Geometry: final body of the model. Coordinates: model frame, mm. Give positions to 0.01 mm unless a question says otherwise; leave off trailing zeros. Write each loop counter-clockwise with the first axis right and the second up, starting at its lowest first coordinate (ties: lowest second). Pieces come first, ordered by that corner, then holes.
Q1. Line query: L1, parallel to Y at x = 2.5, z = 261.5; L2, parallel to Z at x = 1, y = 2; L3, parallel to Z at x = 0.5, y = 1.5. Output: solid intervals per line, ascending.
Q2. Cut plane D-D on y = 71. Return the cut outline in (x, z).
Q3. Cut plane A-A on z = -257. Return the cut outline in (x, y).
Q4. Cut plane B-B on y = 13.5. Return the cut outline in (x, z), plus the area to 3 significant figures.
Q5. Cut plane C-C on x = 3.5. Count the separate pieces of the cut face and the enclosed holes in it, plus the area to 3 significant figures.
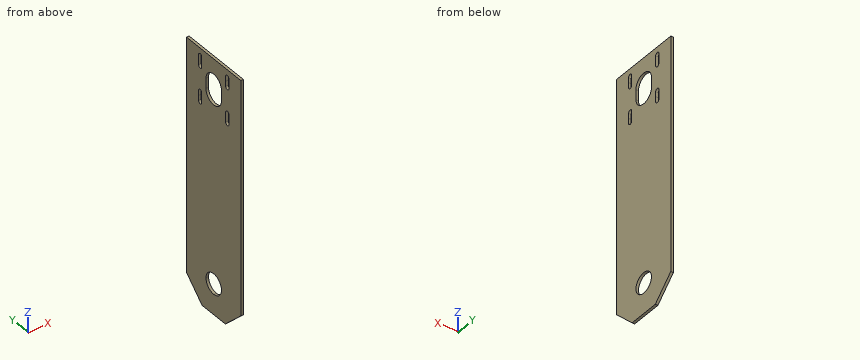
```python
from build123d import *

# Parameters (mm, degrees)
F1_DEPTH = 6.35


# Not quite as in the source:
# - ends of sketch curves that miss each other by under 0.0002 mm in the source are joined


with BuildPart() as f1:
    # F0 (on Right) → F1 (new body)
    with BuildSketch(Plane.YZ):
        Polygon((0, 292.1), (-88.9, 292.1), (-88.9, -292.1), (-38.1, -342.9), (0, -342.9), (38.1, -342.9), (88.9, -292.1), (88.9, 292.1), align=None)
        with BuildLine():
            ThreePointArc((25.4220090151, -266.7011916637), (17.974738209, -284.6694835829), (0, -292.1011821284))
            ThreePointArc((0, -292.1011821284), (-17.9307201788, -248.7328997446), (25.4220090151, -266.7011916637))
        make_face(mode=Mode.SUBTRACT)
        with BuildLine():
            Line((-39.2938236907, 184.15), (-39.2938236907, 171.45))
            Line((-39.2938236907, 171.45), (-39.2938236907, 158.7656303343))
            ThreePointArc((-39.2938236907, 158.7656303343), (-39.2938059227, 158.7578151761), (-39.2938, 158.75))
            ThreePointArc((-39.2938, 158.75), (-44.3355371946, 153.59507064), (-49.6011180661, 158.5211308033))
            ThreePointArc((-49.6011180661, 158.5211308033), (-49.6062, 158.75), (-49.6011180661, 158.9788691967))
            Line((-49.6011180661, 158.9788691967), (-49.6011180661, 171.2211308033))
            ThreePointArc((-49.6011180661, 171.2211308033), (-49.6062, 171.45), (-49.6011180661, 171.6788691967))
            Line((-49.6011180661, 171.6788691967), (-49.6011180661, 183.9211308033))
            ThreePointArc((-49.6011180661, 183.9211308033), (-44.5722759242, 189.3047499492), (-39.2938236907, 184.1656303343))
            ThreePointArc((-39.2938236907, 184.1656303343), (-39.2938059227, 184.1578151761), (-39.2938236907, 184.15))
        make_face(mode=Mode.SUBTRACT)
        with BuildLine():
            ThreePointArc((-39.2963037105, 260.5106642339), (-39.2944259656, 260.4303418705), (-39.2938, 260.35))
            ThreePointArc((-39.2938, 260.35), (-39.2944259656, 260.2696581295), (-39.2963037105, 260.1893357661))
            Line((-39.2963037105, 260.1893357661), (-39.2963037105, 247.8106642339))
            ThreePointArc((-39.2963037105, 247.8106642339), (-39.2944259656, 247.7303418705), (-39.2938, 247.65))
            ThreePointArc((-39.2938, 247.65), (-39.2944259656, 247.5696581295), (-39.2963037105, 247.4893357661))
            ThreePointArc((-39.2963037105, 247.4893357661), (-44.5304520833, 242.4944276843), (-49.6061999953, 247.6502204525))
            Line((-49.6061999953, 247.6502204525), (-49.6056602081, 260.2753926376))
            ThreePointArc((-49.6056602081, 260.2753926376), (-49.6061999953, 260.3502204525), (-49.6056538096, 260.4250482209))
            Line((-49.6056538096, 260.4250482209), (-49.6051185467, 272.9444007144))
            ThreePointArc((-49.6051185467, 272.9444007144), (-44.583133659, 278.2044809505), (-39.2963037105, 273.2106642339))
            ThreePointArc((-39.2963037105, 273.2106642339), (-39.2944259656, 273.1303418705), (-39.2938, 273.05))
            ThreePointArc((-39.2938, 273.05), (-39.2944259656, 272.9696581295), (-39.2963037105, 272.8893357661))
            Line((-39.2963037105, 272.8893357661), (-39.2963037105, 260.5106642339))
        make_face(mode=Mode.SUBTRACT)
        with BuildLine():
            ThreePointArc((-25.4, 228.6), (-17.9605122421, 246.5605122421), (0, 254))
            ThreePointArc((0, 254), (17.9605122421, 246.5605122421), (25.4, 228.6))
            Line((25.4, 228.6), (25.4, 203.2))
            ThreePointArc((25.4, 203.2), (0, 177.8), (-25.4, 203.2))
            Line((-25.4, 203.2), (-25.4, 228.6))
        make_face(mode=Mode.SUBTRACT)
        with BuildLine():
            ThreePointArc((49.6059938769, 171.496104026), (49.606148469, 171.4730522434), (49.6062, 171.45))
            ThreePointArc((49.6062, 171.45), (49.606148469, 171.4269477566), (49.6059938769, 171.403895974))
            Line((49.6059938769, 171.403895974), (49.6059938769, 158.796104026))
            ThreePointArc((49.6059938769, 158.796104026), (49.606148469, 158.7730522434), (49.6062, 158.75))
            ThreePointArc((49.6062, 158.75), (44.4268978801, 153.5938517543), (39.294007016, 158.7962037759))
            Line((39.294007016, 158.7962037759), (39.294007016, 171.4037962241))
            ThreePointArc((39.294007016, 171.4037962241), (39.2938, 171.45), (39.294007016, 171.4962037759))
            Line((39.294007016, 171.4962037759), (39.294007016, 184.1037962241))
            ThreePointArc((39.294007016, 184.1037962241), (44.403846099, 189.3059934307), (49.6059938769, 184.196104026))
            ThreePointArc((49.6059938769, 184.196104026), (49.606148469, 184.1730522434), (49.6062, 184.15))
            ThreePointArc((49.6062, 184.15), (49.606148469, 184.1269477566), (49.6059938769, 184.103895974))
            Line((49.6059938769, 184.103895974), (49.6059938769, 171.496104026))
        make_face(mode=Mode.SUBTRACT)
        with BuildLine():
            ThreePointArc((39.2938, 273.05), (44.45, 278.2062), (49.6062, 273.05))
            Line((49.6062, 273.05), (49.6062, 260.35))
            Line((49.6062, 260.35), (49.6062, 247.65))
            ThreePointArc((49.6062, 247.65), (44.45, 242.4938), (39.2938, 247.65))
            Line((39.2938, 247.65), (39.2938, 260.35))
            Line((39.2938, 260.35), (39.2938, 273.05))
        make_face(mode=Mode.SUBTRACT)
    extrude(amount=F1_DEPTH)


solid = f1.part
```
Data:
1. L1: y = -88.9 to -49.61, -39.3 to 39.29, 49.61 to 88.9
1. L2: z = -342.9 to -292.02, -241.38 to 177.88, 253.92 to 292.1
1. L3: z = -342.9 to -292.06, -241.34 to 177.84, 253.96 to 292.1
2. outline: (0, -310) - (6.35, -310) - (6.35, 292.1) - (0, 292.1) - close
3. outline: (0, -88.9) - (6.35, -88.9) - (6.35, -23.45) - (0, -23.45) - close; (0, 23.5) - (6.35, 23.5) - (6.35, 88.9) - (0, 88.9) - close
4. outline: (0, -342.9) - (6.35, -342.9) - (6.35, -288.23) - (0, -288.23) - close; (0, -245.17) - (6.35, -245.17) - (6.35, 181.68) - (0, 181.68) - close; (0, 250.12) - (6.35, 250.12) - (6.35, 292.1) - (0, 292.1) - close
4. area: 3,320 mm2
5. separate pieces: 1
5. enclosed holes: 6
5. area: 104,000 mm2
